Here's how the part is built. I have some questions about the finished solid (model axes, mm). Face numbers are marked on the shaded views. Round coordinates to 2 decimals unless told otherwise and drop trailing zeros. Loops run counter-clockwise (first coordinate to the right, second up) from the corner with the lowest first, then second, coordinate; pieces in that order, holes last. Notation, with made-up numbers: (17, 18) - (61, 18) arc R23 ccw to (61, 53) - close; hole circle Ø9 at (-24, -25.5). An arc over 180 degrees is marked (long way). Answer as a JSON object with one key per item and string values. Group by question number.
1) I want a section at C-C, the plane x = -10. Please give me the cut outline in (y, z), then the cut area to 3 significant figures.
2) If we mould it in two halves opening along Z, with no side actions, what happens to the marked faces 1 and 2? For each: pulls with the +Z half, pulls with the -Z half, needs draft (parallel to the pull), parting line crosses it, or undercut.
3) If I drill on line 1 along Y through (x, z) = (-0.85, 0); line 2 along Y through (x, z) = (-7.25, 9); line 3 along Z through (x, y) = (-9.25, 17.5), over which ranges is the centre line in solid material (lowest first)? Write a range as [from, to].
4) I want a section at D-D, the plane y = -16. Please give me the cut outline in (x, z), then the cut area to 3 significant figures.
5) I want a section at A-A, the plane y = 32. Please give me the cut outline in (x, z).
6) Will these pins go through, and if not, where does the flat tip stop? P1, Ø2.5, axis at y = 13.5, z = -10, coming from the -X side; P2, Ø1.6, axis at x = -0.5, y = 16.5, coming from the -Z side; P3, Ø0.8, axis at x = -0.5, y = 18, coming from the +Z side; P4, Ø12, axis at y = 20, z = -18.5, coming from the -X side.
7) I want a section at B-B, the plane z = -9. Please give me the cut outline in (x, y), then the cut area to 3 significant figures.
from build123d import *

# Parameters (mm, degrees)
COVER_DISK_OD70_THICKNESS3_W                   = 3
COVER_DISK_OD70_THICKNESS3_H                   = 35
INTEGRAL_START                                 = -11
TWO_INTEGRAL_OD14_PORT_BOSSES_SKETCH_R         = 7
INTEGRAL_PORT_BOSSES_REAR8MM_DEPTH             = 8
SIX_START                                      = -3
SIX_M3_CLEARANCE_HOLES_DIAMETER3P4_P_2_R       = 1.7
SIX_M3_CLEARANCE_HOLES_DIAMETER3P4_PCD64_DEPTH = 3
TWO_START                                      = -11
TWO_G1_8_TAPPING_PILOT_ENVELOPES_DIA_2_R       = 4.4
TWO_G1_8_TAPPING_PILOT_ENVELOPES_DIAMETE_DEPTH = 7
TWO_WATER_PASSAGES_DIAMETER4_SKETCH_R          = 2
TWO_WATER_PASSAGES_DIAMETER4_DEPTH             = 11
INTERNAL_START                                 = -1.5
INTERNAL_BYPASS_STRIP_GROOVE_LENGTH16_WI_DEPTH = 1.5


with BuildPart() as part:
    # Cover disk OD70 thickness3 → One-piece copper cover blank (revolve)
    with BuildSketch(Plane.XY, mode=Mode.PRIVATE) as one_piece_copper_cover_blank_sk:
        with Locations((-1.5, 17.5)):
            Rectangle(COVER_DISK_OD70_THICKNESS3_W, COVER_DISK_OD70_THICKNESS3_H)
    revolve(one_piece_copper_cover_blank_sk.sketch.rotate(Axis((-30, 0, 0), (1, 0, 0)), 90), axis=Axis((-30, 0, 0), (1, 0, 0)))

    # Two integral OD14 port bosses sketch → Integral port bosses rear8mm (add)
    with BuildSketch(Plane(origin=(0, 0, 0), x_dir=(0, 0, -1), z_dir=(1, 0, 0)).offset(INTEGRAL_START)):
        with Locations((-9, 15.588457268)):
            Circle(TWO_INTEGRAL_OD14_PORT_BOSSES_SKETCH_R)
        with Locations((9, 15.588457268)):
            Circle(TWO_INTEGRAL_OD14_PORT_BOSSES_SKETCH_R)
    extrude(amount=INTEGRAL_PORT_BOSSES_REAR8MM_DEPTH)

    # Six M3 clearance holes diameter3p4 P 2 → Six M3 clearance holes diameter3p4 PCD64 (cut)
    with BuildSketch(Plane(origin=(0, 0, 0), x_dir=(0, 0, -1), z_dir=(1, 0, 0)).offset(SIX_START)):
        with Locations((0, 32)):
            Circle(SIX_M3_CLEARANCE_HOLES_DIAMETER3P4_P_2_R)
        with Locations((-27.712812921, 16)):
            Circle(SIX_M3_CLEARANCE_HOLES_DIAMETER3P4_P_2_R)
        with Locations((-27.712812921, -16)):
            Circle(SIX_M3_CLEARANCE_HOLES_DIAMETER3P4_P_2_R)
        with Locations((0, -32)):
            Circle(SIX_M3_CLEARANCE_HOLES_DIAMETER3P4_P_2_R)
        with Locations((27.712812921, -16)):
            Circle(SIX_M3_CLEARANCE_HOLES_DIAMETER3P4_P_2_R)
        with Locations((27.712812921, 16)):
            Circle(SIX_M3_CLEARANCE_HOLES_DIAMETER3P4_P_2_R)
    extrude(amount=SIX_M3_CLEARANCE_HOLES_DIAMETER3P4_PCD64_DEPTH, mode=Mode.SUBTRACT)

    # Two G1-8 tapping pilot envelopes dia 2 → Two G1-8 tapping pilot envelopes diamete (cut)
    with BuildSketch(Plane(origin=(0, 0, 0), x_dir=(0, 0, -1), z_dir=(1, 0, 0)).offset(TWO_START)):
        with Locations((-9, 15.588457268)):
            Circle(TWO_G1_8_TAPPING_PILOT_ENVELOPES_DIA_2_R)
        with Locations((9, 15.588457268)):
            Circle(TWO_G1_8_TAPPING_PILOT_ENVELOPES_DIA_2_R)
    extrude(amount=TWO_G1_8_TAPPING_PILOT_ENVELOPES_DIAMETE_DEPTH, mode=Mode.SUBTRACT)

    # Two water passages diameter4 sketch → Two water passages diameter4 (cut)
    with BuildSketch(Plane(origin=(0, 0, 0), x_dir=(0, 0, -1), z_dir=(1, 0, 0)).offset(TWO_START)):
        with Locations((-9, 15.588457268)):
            Circle(TWO_WATER_PASSAGES_DIAMETER4_SKETCH_R)
        with Locations((9, 15.588457268)):
            Circle(TWO_WATER_PASSAGES_DIAMETER4_SKETCH_R)
    extrude(amount=TWO_WATER_PASSAGES_DIAMETER4_DEPTH, mode=Mode.SUBTRACT)

    # Internal bypass-strip groove length1 2 → Internal bypass-strip groove length16 wi (cut)
    with BuildSketch(Plane(origin=(0, 0, 0), x_dir=(0, 0, -1), z_dir=(1, 0, 0)).offset(INTERNAL_START)):
        with BuildLine():
            Line((1.3, 11.3), (1.3, 24.7))
            ThreePointArc((1.3, 24.7), (0, 26), (-1.3, 24.7))
            Line((-1.3, 24.7), (-1.3, 11.3))
            ThreePointArc((-1.3, 11.3), (0, 10), (1.3, 11.3))
        make_face()
    extrude(amount=INTERNAL_BYPASS_STRIP_GROOVE_LENGTH16_WI_DEPTH, mode=Mode.SUBTRACT)


solid = part.part
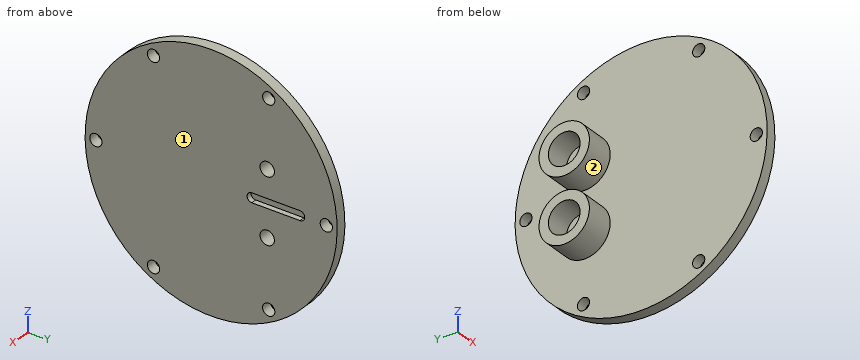
Outcome:
{
 "1": {"outline": "circle Ø14 at (15.59, -9); circle Ø14 at (15.59, 9); hole circle Ø8.8 at (15.59, -9); hole circle Ø8.8 at (15.59, 9)", "area": "186 mm^2"},
 "2": {"face 1": "needs draft", "face 2": "undercut"},
 "3": {"line 1": "[-35, -33.7], [-30.3, 10], [26, 30.3], [33.7, 35]", "line 2": "[8.59, 11.19], [19.99, 22.59]", "line 3": "[-15.73, -12.96], [-5.04, -2.27], [2.27, 5.04], [12.96, 15.73]"},
 "4": {"outline": "(-3, -31.13) - (0, -31.13) - (0, -29.41) - (-3, -29.41) - close; (-3, -26.01) - (0, -26.01) - (0, 26.01) - (-3, 26.01) - close; (-3, 29.41) - (0, 29.41) - (0, 31.13) - (-3, 31.13) - close", "area": "166 mm^2"},
 "5": {"outline": "(-3, -14.18) - (0, -14.18) - (0, -1.7) - (-3, -1.7) - close; (-3, 1.7) - (0, 1.7) - (0, 14.18) - (-3, 14.18) - close"},
 "6": {"P1": "x = -4", "P2": "z = -31.28", "P3": "z = 30.25", "P4": "x = -11"},
 "7": {"outline": "(-11, 8.59) - (-3, 8.59) - (-3, -33.82) - (0, -33.82) - (0, 13.59) - (-4, 13.59) - (-4, 11.19) - (-11, 11.19) - close; (-11, 19.99) - (-4, 19.99) - (-4, 17.59) - (0, 17.59) - (0, 33.82) - (-3, 33.82) - (-3, 22.59) - (-11, 22.59) - close", "area": "237 mm^2"}
}
